Source: CAD feature listing. Evaluate the final solid. Frame: model axes, mm. Face numbers are marked on the shaded views. A direction names the side the tool comes from. Round coordinates to 2 decimals unless told otherwise and drop trailing zeros. Write each loop counter-clockwise with the first axis right and the second up, starting at its lowest first coordinate (ties: lowest second). Pieces come first, ordered by that corner, then holes. Notation, with made-up numbers: (11, 74) -> (29, 74) arc R26 cw to (29, 95) -> close; hole circle Ø9 at (68.5, 89.25). An arc over 180 degrees is marked (long way). Put each result on its own line as item: value.
```python
from build123d import *

# Parameters (mm, degrees)
SM_BASE_FLANGE_1_DEPTH = 20.5
FILLET_1_R             = 20.5
MM_1_D                 = 3
MM_1_DEPTH             = 7.5
MM_1_TIP               = 0.901290929
SKETCH_10_R            = 1.75
CUT_EXTRUDE_1_DEPTH    = 10
CUT_EXTRUDE_2_DEPTH    = 10


# Sheet-metal steps are written as plain solids
with BuildPart() as part:
    # Sketch 1 → 基体-法兰1 (new, symmetric)
    with BuildSketch(Plane.XY):
        with BuildLine():
            Line((0, 0), (0, 38.7634))
            ThreePointArc((0, 38.7634), (0.655084973, 40.344915027), (2.2366, 41))
            Line((2.2366, 41), (45, 41))
            Line((45, 41), (45, 39.5))
            Line((45, 39.5), (2.2366, 39.5))
            ThreePointArc((2.2366, 39.5), (1.715745145, 39.284254855), (1.5, 38.7634))
            Line((1.5, 38.7634), (1.5, 0))
            Line((1.5, 0), (0, 0))
        make_face()
    extrude(amount=SM_BASE_FLANGE_1_DEPTH, both=True)

    # 圆角1
    fillet_1_edges = [part.edges().sort_by_distance(p)[0] for p in [
        (45, 40.25, -20.5),
        (45, 40.25, 20.5),
    ]]
    fillet(fillet_1_edges, radius=FILLET_1_R - 0.0001)  # a hair under: the kernel refuses the full size

    # 大小mm 暗销孔1
    with Locations(Plane(origin=(0, 41, 0), x_dir=(1, 0, 0), z_dir=(0, 1, 0))):
        with Locations((24.087127043, 15.261627687), (37.923393759, 7.75), (37.923393759, -7.75), (24.5, -15.5), (11.076606241, -7.75), (11.076606241, 7.75)):
            Hole(MM_1_D / 2, depth=MM_1_DEPTH)
            with Locations((0, 0, -(MM_1_DEPTH + MM_1_TIP / 2))):  # 118° drill point
                Cone(0, MM_1_D / 2, MM_1_TIP, mode=Mode.SUBTRACT)

    # 草图10 → 切除-拉伸1 (cut)
    with BuildSketch(Plane.ZY):
        with Locations((-15, 32)):
            Circle(SKETCH_10_R)
        with Locations((15, 32)):
            Circle(SKETCH_10_R)
        with Locations((15, 8)):
            Circle(SKETCH_10_R)
        with Locations((-15, 8)):
            Circle(SKETCH_10_R)
    extrude(amount=-CUT_EXTRUDE_1_DEPTH, mode=Mode.SUBTRACT)

    # 草图11 → 切除-拉伸2 (cut)
    with BuildSketch(Plane.XZ.offset(-39.5)):
        with BuildLine():
            Line((33, -6.25), (13, -6.25))
            ThreePointArc((13, -6.25), (6.75, 0), (13, 6.25))
            Line((13, 6.25), (33, 6.25))
            ThreePointArc((33, 6.25), (39.25, 0), (33, -6.25))
        make_face()
    extrude(amount=-CUT_EXTRUDE_2_DEPTH, mode=Mode.SUBTRACT)


solid = part.part
```
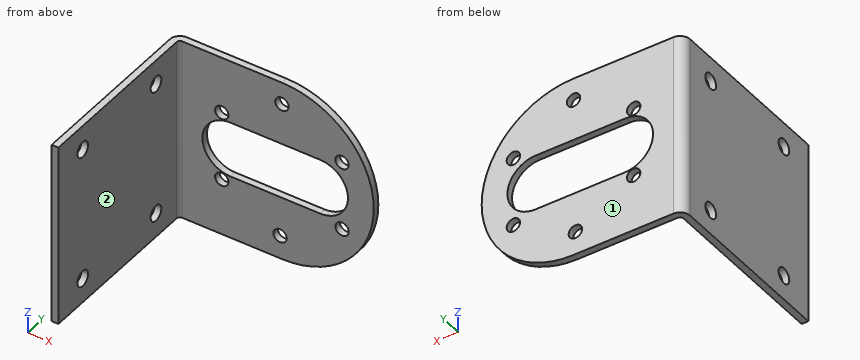
Q1. Cut plane D-D on z = 15.5. Output: boundary loops of the cut face in (x, y).
Ans:
outline: (0, 0) -> (1.5, 0) -> (1.5, 6.32) -> (0, 6.32) -> close; (0, 9.68) -> (1.5, 9.68) -> (1.5, 30.32) -> (0, 30.32) -> close; (0, 33.68) -> (1.5, 33.68) -> (1.5, 38.76) arc R0.74 cw to (2.24, 39.5) -> (23, 39.5) -> (23, 41) -> (2.24, 41) arc R2.24 ccw to (0, 38.76) -> close; (26, 39.5) -> (37.92, 39.5) -> (37.92, 41) -> (26, 41) -> close
Q2. Cut plane C-C on x = 35. Output: boundary loops of the cut face in (y, z), and give its area (3 significant figures).
Ans:
outline: (39.5, -17.61) -> (41, -17.61) -> (41, -5.92) -> (39.5, -5.92) -> close; (39.5, 5.92) -> (41, 5.92) -> (41, 17.61) -> (39.5, 17.61) -> close
area: 35.1 mm^2
Q3. Material intervals for line 1 (Y direction, x = 1, z = 15); line 2 (X direction, y = 11, z = -9); line 3 (Y direction, x = 31.5, z = 17), sorted ascending. Write a range as [from, to].
Ans:
line 1: y = [0, 6.25], [9.75, 30.25], [33.75, 40.63]
line 2: x = [0, 1.5]
line 3: y = [39.5, 41]
Q4. Pin query (flat end, axial travel): pin 1 (11.5 mm diameter, centred on y = 24.5, z = 4.5, fed in from +X); pin 2 (8 mm diameter, centred on y = 22, z = 7, fed in from -X); pin 3 (12 mm diameter, centred on x = 12, y = 14, fed in from -Z); pin 4 (2 mm diameter, centred on x = 19.5, z = 14.5, fed in from -Y). Return the tip coordinate at first contact, or that it passes through.
Ans:
pin 1: stops at x = 1.5
pin 2: stops at x = 0
pin 3: passes through
pin 4: stops at y = 39.5
Q5. Cut plane A-A on z = -8.5. Output: boundary loops of the cut face in (x, y), and give its area (3 significant figures).
Ans:
outline: (0, 0) -> (1.5, 0) -> (1.5, 38.76) arc R0.74 cw to (2.24, 39.5) -> (9.78, 39.5) -> (9.78, 41) -> (2.24, 41) arc R2.24 ccw to (0, 38.76) -> close; (12.38, 39.5) -> (36.62, 39.5) -> (36.62, 41) -> (12.38, 41) -> close; (39.22, 39.5) -> (43.15, 39.5) -> (43.15, 41) -> (39.22, 41) -> close
area: 115 mm^2
Q6. Cut plane B-B on y = 7. Output: boundary loops of the cut face in (x, z), and give its area (3 significant figures).
Ans:
outline: (0, -20.5) -> (1.5, -20.5) -> (1.5, -16.44) -> (0, -16.44) -> close; (0, -13.56) -> (1.5, -13.56) -> (1.5, 13.56) -> (0, 13.56) -> close; (0, 16.44) -> (1.5, 16.44) -> (1.5, 20.5) -> (0, 20.5) -> close
area: 52.9 mm^2
Q7. Reachability of the marked faces 1 and 2 from +Z, -Z, +X, -X, +Y, -Y: full face, straight path, thin tool, end or side. Return the list, or none.
Ans:
face 1: +Z, -Z, +X, -X, +Y
face 2: +Z, -Z, +X, -Y
